from build123d import *

# Parameters (mm, degrees)
F1_DEPTH = 60
F2_R     = 5
F3_SIZE  = 5
F4_R     = 19.052839
F5_DEPTH = 30


with BuildPart() as f1:
    # F0 (on Front) → F1 (new body)
    with BuildSketch(Plane.XZ):
        with BuildLine():
            Line((36.56146, 58.775878), (-13.43854, 58.775878))
            ThreePointArc((-13.43854, 58.775878), (-31.116209, 51.453547), (-38.43854, 33.775878))
            Line((-38.43854, 33.775878), (-38.43854, -16.224122))
            ThreePointArc((-38.43854, -16.224122), (-31.116209, -33.901792), (-13.43854, -41.224122))
            Line((-13.43854, -41.224122), (36.56146, -41.224122))
            ThreePointArc((36.56146, -41.224122), (54.23913, -33.901792), (61.56146, -16.224122))
            Line((61.56146, -16.224122), (61.56146, 33.775878))
            ThreePointArc((61.56146, 33.775878), (54.23913, 51.453547), (36.56146, 58.775878))
        make_face()
    extrude(amount=F1_DEPTH)

    # F2
    f2_edges = [f1.edges().sort_by_distance(p)[0] for p in [
        (11.56146, -60, 58.775878),
        (-31.116209, -60, 51.453547),
        (-38.43854, -60, 8.775878),
        (-31.116209, -60, -33.901792),
        (11.56146, -60, -41.224122),
        (54.23913, -60, -33.901792),
        (61.56146, -60, 8.775878),
        (54.23913, -60, 51.453547),
    ]]
    fillet(f2_edges, radius=F2_R)

    # F3
    f3_edges = [f1.edges().sort_by_distance(p)[0] for p in [
        (11.56146, 0, 58.775878),
        (-31.116209, 0, 51.453547),
        (-38.43854, 0, 8.775878),
        (-31.116209, 0, -33.901792),
        (11.56146, 0, -41.224122),
        (54.23913, 0, -33.901792),
        (61.56146, 0, 8.775878),
        (54.23913, 0, 51.453547),
    ]]
    chamfer(f3_edges, length=F3_SIZE)

    # F4 (on face) → F5 (cut)
    with BuildSketch(Plane.XZ.offset(60)):
        with Locations((9.132151, 8.183358)):
            Circle(F4_R)
    extrude(amount=-F5_DEPTH, mode=Mode.SUBTRACT)


solid = f1.part
The listing builds one solid part. Answer for the finished solid, in the listing's coordinates (mm). A direction names the side the tool comes from. Coordinates: 2 decimals unless noted, no trailing zeros. Write each loop counter-clockwise with the first axis right and the second up, starting at its lowest first coordinate (ties: lowest second). Pieces come first, ordered by that corner, then holes. Notation, with made-up numbers: M -15.75,-4.5 L 33.25,-4.5 A20 ccw 33.25,24.5 Z; hole C 10.5,60.25 d8. An arc over 180 degrees is marked long. Put each result on its own line as item: value. Start each with the question number.
1. A cutting plane is placed at A-A on y = -47. Write down the section's boundary in (x, z).
2. Consider line 1 (X direction, y = -56, z = 3.5); line 2 (Y direction, x = 27.5, z = 10.5); line 3 (X direction, y = -36, z = 18.5). Determine where each line is inside the solid, lowest interval first. Write a range as from..to.
3. Flat-ended cylindrical pins translate along their axes: P1, Ø2, axis at x = -16.5, y = -36.5, coming from the +Z side; P2, Ø19, axis at x = 5.5, z = 6, coming from the -Y side; P3, Ø12, axis at y = -51.5, z = 48, coming from the -X side. Find the tip coordinate at first contact, or state that the pin passes through.
4. A cutting plane is placed at B-B on y = -10. Write down the section's boundary in (x, z), then the cut area to 3 significant figures.
5. For a pull along Z with two mould halves and no side action, classify faces 1 (the flat face through (9, -30, 8)), 2 (the cylindrical face through (-37.01, -58.5, 8.43)), 3 (the cylindrical face through (11.911, -58.496, -39.798)), 4 (the cylindrical face through (54.43, -29.65, 51.26)) as pulls with the +Z half, pulls with the -Z half, needs draft (parallel to the pull), parting line crosses it, or undercut.
6. A cutting plane is placed at C-C on z = 24. Write down the section's boundary in (x, y), then the cut area to 3 significant figures.
7. A cutting plane is placed at D-D on x = 2. Write down the section's boundary in (y, z).
8. Which of the six approach directions +Z, -Z, +X, -X, +Y, -Y give full straight-line access (tool end or side, diameter ignored) to faces 5 (the flat face through (-35.9, -2.46, 9.13)), 6 (the cylindrical face through (-5.99, -45.21, -3.41))?
Resolved:
1. outline: M -38.44,-16.22 A25 ccw -13.44,-41.22 L 36.56,-41.22 A25 ccw 61.56,-16.22 L 61.56,33.78 A25 ccw 36.56,58.78 L -13.44,58.78 A25 ccw -38.44,33.78 Z; hole C 9.13,8.18 d38.11
2. line 1: x = -38.34..-9.34, 27.6..61.46
2. line 2: y = -30..0
2. line 3: x = -38.44..-6.89, 25.15..61.56
3. P1: stops at z = 58.69
3. P2: stops at y = -30
3. P3: stops at x = -37.05
4. outline: M -38.44,-16.22 A25 ccw -13.44,-41.22 L 36.56,-41.22 A25 ccw 61.56,-16.22 L 61.56,33.78 A25 ccw 36.56,58.78 L -13.44,58.78 A25 ccw -38.44,33.78 Z
4. area: 9,460 mm2
5. face 1: undercut
5. face 2: needs draft
5. face 3: pulls with the -Z half
5. face 4: pulls with the +Z half
6. outline: M -38.44,-55 A5 ccw -33.44,-60 L -1.49,-60 L -1.49,-30 L 19.75,-30 L 19.75,-60 L 56.56,-60 A5 ccw 61.56,-55 L 61.56,-5 L 56.56,0 L -33.44,0 L -38.44,-5 Z
6. area: 5,330 mm2
7. outline: M -60,-36.22 A5 ccw -55,-41.22 L -5,-41.22 L 0,-36.22 L 0,53.78 L -5,58.78 L -55,58.78 A5 ccw -60,53.78 L -60,25.85 L -30,25.85 L -30,-9.48 L -60,-9.48 Z
8. face 5: +Z, -Z, -X, +Y
8. face 6: -Y
